Work out the finished part from the listing and answer in its coordinate system (mm). Coordinates: 2 decimals unless noted, no trailing zeros. Write each loop counter-clockwise with the first axis right and the second up, starting at its lowest first coordinate (ties: lowest second). Pieces come first, ordered by that corner, then holes. Notation, with made-up numbers: (-18, -11) - (22, -11) arc R26 ccw to (22, 7) - close; hole circle Ø11 at (12.5, -20.75). An arc over 180 degrees is marked (long way). One line per item, written item: value.
```python
from build123d import *

# Parameters (mm, degrees)
SKETCH1_W           = 50
SKETCH1_H           = 170
SKETCH1_R           = 5
SKETCH1_W_2         = 15
SKETCH1_H_2         = 5
BOSS_EXTRUDE1_DEPTH = 5


with BuildPart() as part:
    # Sketch1 → Boss-Extrude1 (new body)
    with BuildSketch(Plane.XY):
        with Locations((-17.719310928, 76.759780871)):
            Rectangle(SKETCH1_W, SKETCH1_H)
        with Locations((-15.705505676, 29.999739242)):
            Circle(SKETCH1_R, mode=Mode.SUBTRACT)
        with Locations((-15.413646235, 99.999739242)):
            Circle(SKETCH1_R, mode=Mode.SUBTRACT)
        with Locations((-31.219310928, 9.449835726)):
            Rectangle(SKETCH1_W_2, SKETCH1_H_2, mode=Mode.SUBTRACT)
        with Locations((-31.219310928, 86.716581053)):
            Rectangle(SKETCH1_W_2, SKETCH1_H_2, mode=Mode.SUBTRACT)
        with Locations((-4.219310928, 86.716581053)):
            Rectangle(SKETCH1_W_2, SKETCH1_H_2, mode=Mode.SUBTRACT)
        with Locations((-4.219310928, 9.449835726)):
            Rectangle(SKETCH1_W_2, SKETCH1_H_2, mode=Mode.SUBTRACT)
    extrude(amount=BOSS_EXTRUDE1_DEPTH)


solid = part.part
```
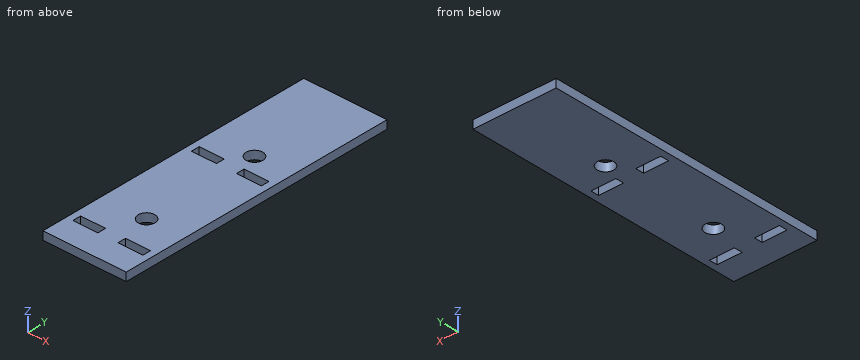
Item 1: Section C-C, the plane z = 2.95 is taken. Determine the outline of the cut face in (x, y).
Evaluation:
outline: (-42.72, -8.24) - (7.28, -8.24) - (7.28, 161.76) - (-42.72, 161.76) - close; hole (-38.72, 6.95) - (-23.72, 6.95) - (-23.72, 11.95) - (-38.72, 11.95) - close; hole (-38.72, 84.22) - (-23.72, 84.22) - (-23.72, 89.22) - (-38.72, 89.22) - close; hole circle Ø10 at (-15.71, 30); hole circle Ø10 at (-15.41, 100); hole (-11.72, 6.95) - (3.28, 6.95) - (3.28, 11.95) - (-11.72, 11.95) - close; hole (-11.72, 84.22) - (3.28, 84.22) - (3.28, 89.22) - (-11.72, 89.22) - close
Item 2: Section B-B, the plane y = 33.5 is taken. Determine the outline of the cut face in (x, z), then the cut area to 3 significant figures.
Evaluation:
outline: (-42.72, 0) - (-19.28, 0) - (-19.28, 5) - (-42.72, 5) - close; (-12.14, 0) - (7.28, 0) - (7.28, 5) - (-12.14, 5) - close
area: 214 mm2
Item 3: Consider probe 1 along Y at (x, z) = (-1, 4.45); probe 2 along Y at (x, z) = (-14.5, 2.4); probe 3 along X at (y, z) = (28, 1.8). Determine where each line is inside the solid, lowest interval first.
Evaluation:
probe 1: y = -8.24 to 6.95, 11.95 to 84.22, 89.22 to 161.76
probe 2: y = -8.24 to 25.15, 34.85 to 95.08, 104.92 to 161.76
probe 3: x = -42.72 to -20.29, -11.12 to 7.28
Item 4: Section D-D, the plane x = -16.5 is taken. Determine the outline of the cut face in (y, z).
Evaluation:
outline: (-8.24, 0) - (25.06, 0) - (25.06, 5) - (-8.24, 5) - close; (34.94, 0) - (95.12, 0) - (95.12, 5) - (34.94, 5) - close; (104.88, 0) - (161.76, 0) - (161.76, 5) - (104.88, 5) - close
Item 5: Section A-A, the plane x = -31 is taken. Determine the outline of the cut face in (y, z).
Evaluation:
outline: (-8.24, 0) - (6.95, 0) - (6.95, 5) - (-8.24, 5) - close; (11.95, 0) - (84.22, 0) - (84.22, 5) - (11.95, 5) - close; (89.22, 0) - (161.76, 0) - (161.76, 5) - (89.22, 5) - close
